Design review of the part built by this model. Coordinates are the model's own, in mm. Coordinates: 2 decimals unless noted, no trailing zeros. Write each loop counter-clockwise with the first axis right and the second up, starting at its lowest first coordinate (ties: lowest second). Pieces come first, ordered by that corner, then holes.
Q1. Add section B-B, the plane z = -14. Give the boundary of the cut face in (x, y).
Q2. Add section A-A, the plane x = 433. Give the boundary of the cut face in (y, z).
Q3. To check wall thickness, follow probe 1 along Z at (x, y) = (126, 6); probe 2 along Y at (x, z) = (346.5, -10); probe 3 along Z at (x, y) = (323, -12.5). State the ranges of each line that lie inside material, in increasing order.
Q4. Clearance check with a flat-ended pin moving along its axis: pin 1 Ø5 at (x, y) = (185, -0.5) entering from -Z (3 decimals). State where the tip first meets the part, or that it passes through.
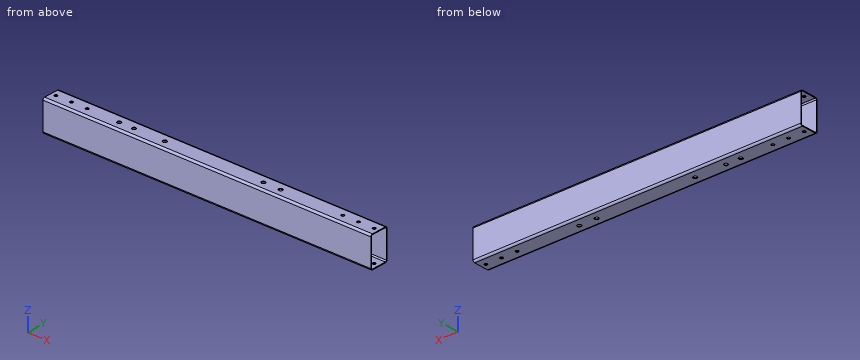
from build123d import *

# Parameters (mm, degrees)
TUBO_RETANGULAR_50_X_30_X_2_6_1_DEPTH = 532
ESBO_O2_R                             = 2.5
CORTE_EXTRUS_O1_DEPTH                 = 535.554955079
ESBO_O3_R                             = 3.25
CORTE_EXTRUS_O2_DEPTH                 = 535.554955079
ESBO_O4_R                             = 3.25
CORTE_EXTRUS_O3_DEPTH                 = 535.554955079


with BuildPart() as part:
    # Sketch1 → Tubo retangular 50 X 30 X 2.6(1) (new body)
    with BuildSketch(Plane.YZ):
        with BuildLine():
            Line((-12, -25), (12, -25))
            ThreePointArc((12, -25), (14.121320344, -24.121320344), (15, -22))
            Line((15, -22), (15, 22))
            ThreePointArc((15, 22), (14.121320344, 24.121320344), (12, 25))
            Line((12, 25), (-12, 25))
            ThreePointArc((-12, 25), (-14.121320344, 24.121320344), (-15, 22))
            Line((-15, 22), (-15, -22))
            ThreePointArc((-15, -22), (-14.121320344, -24.121320344), (-12, -25))
        make_face()
        with BuildLine():
            Line((-12, -23.8), (12, -23.8))
            ThreePointArc((12, -23.8), (13.272792206, -23.272792206), (13.8, -22))
            Line((13.8, -22), (13.8, 22))
            ThreePointArc((13.8, 22), (13.272792206, 23.272792206), (12, 23.8))
            Line((12, 23.8), (-12, 23.8))
            ThreePointArc((-12, 23.8), (-13.272792206, 23.272792206), (-13.8, 22))
            Line((-13.8, 22), (-13.8, -22))
            ThreePointArc((-13.8, -22), (-13.272792206, -23.272792206), (-12, -23.8))
        make_face(mode=Mode.SUBTRACT)
    extrude(amount=TUBO_RETANGULAR_50_X_30_X_2_6_1_DEPTH)

    # Esboço2 → Corte-extrusão1 (cut, through all)
    with BuildSketch(Plane(origin=(0, 0, -25), x_dir=(-1, 0, 0), z_dir=(0, 0, -1))):
        with Locations((-58.5, 0)):
            Circle(ESBO_O2_R)
        with Locations((-33.1, 0)):
            Circle(ESBO_O2_R)
        with Locations((-7.7, 0)):
            Circle(ESBO_O2_R)
        with Locations(Location((-524.3, 0, 0), (0, 0, 180))):
            Circle(ESBO_O2_R)
        with Locations(Location((-498.9, 0, 0), (0, 0, 180))):
            Circle(ESBO_O2_R)
        with Locations(Location((-473.5, 0, 0), (0, 0, 180))):
            Circle(ESBO_O2_R)
    extrude(amount=-CORTE_EXTRUS_O1_DEPTH, mode=Mode.SUBTRACT)

    # Esboço3 → Corte-extrusão2 (cut, through all)
    with BuildSketch(Plane(origin=(0, 0, -25), x_dir=(-1, 0, 0), z_dir=(0, 0, -1))):
        with Locations((-185, -0.5)):
            Circle(ESBO_O3_R)
        with Locations((-111, -0.5)):
            Circle(ESBO_O3_R)
        with Locations((-373, -0.5)):
            Circle(ESBO_O3_R)
    extrude(amount=-CORTE_EXTRUS_O2_DEPTH, mode=Mode.SUBTRACT)

    # Esboço4 → Corte-extrusão3 (cut, through all)
    with BuildSketch(Plane(origin=(0, 0, -25), x_dir=(-1, 0, 0), z_dir=(0, 0, -1))):
        with Locations((-345, -0.5)):
            Circle(ESBO_O4_R)
        with Locations((-135, -0.5)):
            Circle(ESBO_O4_R)
    extrude(amount=-CORTE_EXTRUS_O3_DEPTH, mode=Mode.SUBTRACT)


solid = part.part
Here are the results:
1. outline: (0, -15) - (532, -15) - (532, -13.8) - (0, -13.8) - close; (0, 13.8) - (532, 13.8) - (532, 15) - (0, 15) - close
2. outline: (-15, -22) arc R3 ccw to (-12, -25) - (12, -25) arc R3 ccw to (15, -22) - (15, 22) arc R3 ccw to (12, 25) - (-12, 25) arc R3 ccw to (-15, 22) - close; hole (-13.8, -22) arc R1.8 ccw to (-12, -23.8) - (12, -23.8) arc R1.8 ccw to (13.8, -22) - (13.8, 22) arc R1.8 ccw to (12, 23.8) - (-12, 23.8) arc R1.8 ccw to (-13.8, 22) - close
3. probe 1: z = -25 to -23.8, 23.8 to 25
3. probe 2: y = -15 to -13.8, 13.8 to 15
3. probe 3: z = -24.96 to -23.73, 23.73 to 24.96
4. pin 1: passes through
